CAD build for the part. Positions are in the model's coordinates, mm. A direction names the side the tool comes from. Round coordinates to 2 decimals unless told otherwise and drop trailing zeros. Loops run counter-clockwise (first coordinate to the right, second up) from the corner with the lowest first, then second, coordinate; pieces in that order, holes last. Notation, with made-up numbers: M 15.25,61 L 74.25,61 A34 ccw 74.25,95 Z; hole C 85,29 d2. An arc over 180 degrees is marked long. Put each result on its own line as item: value. Start each with the question number.
from build123d import *

# Parameters (mm, degrees)
F0_W     = 76.2
F0_H     = 76.2
F1_DEPTH = 3.81
F2_W     = 61.9252
F2_H     = 73.025
F3_DEPTH = 1.905
F4_W     = 6.35
F4_H     = 50.8
F5_DEPTH = 25.4
F7_DEPTH = 25.4
F8_W     = 50.8
F8_H     = 5.08
F9_DEPTH = 25.4


with BuildPart() as f1:
    # F0 (on Top) → F1 (new body)
    with BuildSketch(Plane.XY):
        Rectangle(F0_W, F0_H)
    extrude(amount=F1_DEPTH)

    # F2 (on face) → F3 (cut)
    with BuildSketch(Plane.XY.offset(3.81)):
        Rectangle(F2_W, F2_H)
    extrude(amount=-F3_DEPTH, mode=Mode.SUBTRACT)

    # F4 (on face) → F5 (join)
    with BuildSketch(Plane.XY.offset(1.905)):
        Rectangle(F4_W, F4_H)
    extrude(amount=F5_DEPTH)

    # F6 (on face) → F7 (cut)
    with BuildSketch(Plane.YZ.offset(3.175)):
        with BuildLine():
            ThreePointArc((15.24, 9.525), (20.32, 14.605), (15.24, 19.685))
            Line((15.24, 19.685), (-15.24, 19.685))
            ThreePointArc((-15.24, 19.685), (-20.32, 14.605), (-15.24, 9.525))
            Line((-15.24, 9.525), (15.24, 9.525))
        make_face()
    extrude(amount=-F7_DEPTH, mode=Mode.SUBTRACT)

    # F8 (on face) → F9 (cut)
    with BuildSketch(Plane.YZ.offset(3.175)):
        with Locations((0, 24.765)):
            Rectangle(F8_W, F8_H)
    extrude(amount=-F9_DEPTH, mode=Mode.SUBTRACT)


solid = f1.part
(1) Cut at A-A on y = 14. List the corners of the cut face in (x, z) (3 decimals).
(2) Mould opens along Y. For faces 1 (the flat face through (-1, 38.1, 2)), 2 (the flat face through (-1, -38.1, 2)), 3 (the flat face through (-1, 1, 0)), 4 (the flat face through (-30.963, -1, 3)) say: +Y half, -Y half, draft (parallel to the pull), parting line (faces both ways), or undercut.
(3) Cut at D-D on z = 6.75. List the corners of the cut face in (x, y) (3 decimals), and give its area (3 significant figures).
(4) Tool access for faces 5 (the flat face through (0, 0, 22.225)), 6 (the flat face through (-3.175, 0, 7)), 7 (the cylindrical face through (0.04, 20.32, 14.49)): list every direction of +Z, -Z, +X, -X, +Y, -Y with a clear straight run to the whole face (end or side of a thin tool).
(5) Flat gauge pins, fed straight in: pin 1 Ø10 at (y, z) = (-25, 17.5) entering from -X (3 decimals); pin 2 Ø1.9 at (x, z) = (-1, 15.5) entering from -Y; pin 3 Ø4 at (y, z) = (-2, 19.5) entering from +X (3 decimals); pin 4 Ø5 at (y, z) = (-3.5, 15) entering from +X. Where does each tip first touch, or does it go through?
(6) Cut at B-B on z = 11.25. List the corners of the cut face in (x, y) (1 decimal).
(7) Drill centre lines: line 1 along Z through (x, y) = (26, -10) (3 decimals); line 2 along X through (y, z) = (-14, 21.25) (3 decimals); line 3 along Z through (x, y) = (-0.5, -16) (3 decimals). Where is each one in solid material? Low to high.
(8) Cut at C-C on x = 0.5. List the corners of the cut face in (y, z) (1 decimal).
Taken from the geometry:
1. outline: M -38.1,0 L 38.1,0 L 38.1,3.81 L 30.963,3.81 L 30.963,1.905 L 3.175,1.905 L 3.175,9.525 L -3.175,9.525 L -3.175,1.905 L -30.963,1.905 L -30.963,3.81 L -38.1,3.81 Z; M -3.175,19.685 L 3.175,19.685 L 3.175,22.225 L -3.175,22.225 Z
2. face 1: +Y half
2. face 2: -Y half
2. face 3: draft
2. face 4: undercut
3. outline: M -3.175,-25.4 L 3.175,-25.4 L 3.175,25.4 L -3.175,25.4 Z
3. area: 323 mm2
4. face 5: +Z, +X, -X, +Y, -Y
4. face 6: +Z
4. face 7: +X, -X
5. pin 1: x = -3.175
5. pin 2: y = -25.4
5. pin 3: x = 3.175
5. pin 4: through
6. outline: M -3.2,-25.4 L 3.2,-25.4 L 3.2,-19.1 L -3.2,-19.1 Z; M -3.2,19.1 L 3.2,19.1 L 3.2,25.4 L -3.2,25.4 Z
7. line 1: 0 to 1.905
7. line 2: -3.175 to 3.175
7. line 3: 0 to 9.582, 19.628 to 22.225
8. outline: M -38.1,0 L 38.1,0 L 38.1,3.8 L 36.5,3.8 L 36.5,1.9 L 25.4,1.9 L 25.4,22.2 L -25.4,22.2 L -25.4,1.9 L -36.5,1.9 L -36.5,3.8 L -38.1,3.8 Z; hole M -15.2,9.5 L 15.2,9.5 A5.1 ccw 15.2,19.7 L -15.2,19.7 A5.1 ccw Z
